```python
from build123d import *

# Parameters (mm, degrees)
SKETCH1_W           = 178
SKETCH1_H           = 104
SKETCH1_W_2         = 72
SKETCH1_H_2         = 68
BOSS_EXTRUDE1_DEPTH = 1.2
BOSS_EXTRUDE2_DEPTH = 5
SKETCH3_W           = 112
SKETCH3_H           = 10
BOSS_EXTRUDE3_DEPTH = 0.8
SKETCH4_W           = 10
SKETCH4_H           = 10
BOSS_EXTRUDE4_DEPTH = 2.8
SKETCH5_W           = 6
SKETCH5_H           = 2
CUT_EXTRUDE1_DEPTH  = 10
SKETCH6_W           = 10
SKETCH6_H           = 7.8
BOSS_EXTRUDE5_DEPTH = 6
FILLET1_R           = 10
FILLET2_R           = 6
SKETCH7_R           = 1.5
CUT_EXTRUDE2_DEPTH  = 4
FILLET3_R           = 3
SKETCH8_W           = 3
SKETCH8_H           = 10
BOSS_EXTRUDE6_DEPTH = 2.8
FILLET4_R           = 3
SKETCH9_W           = 10
SKETCH9_H           = 78
BOSS_EXTRUDE7_DEPTH = 2
BOSS_EXTRUDE8_DEPTH = 1.2


with BuildPart() as part:
    # Sketch1 → Boss-Extrude1 (new body)
    with BuildSketch(Plane(origin=(0, 0, 0), x_dir=(1, 0, 0), z_dir=(0, 1, 0))):
        with Locations((89, 52)):
            Rectangle(SKETCH1_W, SKETCH1_H)
        with Locations((126, 54)):
            Rectangle(SKETCH1_W_2, SKETCH1_H_2, mode=Mode.SUBTRACT)
        with Locations((44, 54)):
            Rectangle(SKETCH1_W_2, SKETCH1_H_2, mode=Mode.SUBTRACT)
    extrude(amount=BOSS_EXTRUDE1_DEPTH)

    # Sketch2 → Boss-Extrude2 (add)
    with BuildSketch(Plane(origin=(0, 0, -104), x_dir=(-1, 0, 0), z_dir=(0, 0, -1))):
        Polygon((-151, 0), (-148, 0), (-148, -2), (-144, -2), (-144, 0), (-141, 0), (-141, -4), (-144, -4), (-148, -4), (-151, -4), align=None)
    boss_extrude2 = extrude(amount=-BOSS_EXTRUDE2_DEPTH)

    # Mirror1: Boss-Extrude2 across plane
    add(boss_extrude2.mirror(Plane.ZY.offset(-78.75)))

    # Sketch3 → Boss-Extrude3 (add)
    with BuildSketch(Plane.XZ):
        with Locations((66, -10.2)):
            Rectangle(SKETCH3_W, SKETCH3_H)
    extrude(amount=BOSS_EXTRUDE3_DEPTH)

    # Sketch4 → Boss-Extrude4 (add)
    with BuildSketch(Plane.XZ):
        with Locations((5, -10.2)):
            Rectangle(SKETCH4_W, SKETCH4_H)
    extrude(amount=BOSS_EXTRUDE4_DEPTH)

    # Sketch5 → Cut-Extrude1 (cut)
    with BuildSketch(Plane.ZY):
        with Locations((-10.2, -1)):
            Rectangle(SKETCH5_W, SKETCH5_H)
    extrude(amount=-CUT_EXTRUDE1_DEPTH, mode=Mode.SUBTRACT)

    # Sketch6 → Boss-Extrude5 (add)
    with BuildSketch(Plane(origin=(0, 0, -104), x_dir=(-1, 0, 0), z_dir=(0, 0, -1))):
        with Locations((-89.25, -3.9)):
            Rectangle(SKETCH6_W, SKETCH6_H)
    extrude(amount=-BOSS_EXTRUDE5_DEPTH)

    # Fillet1
    # the kernel refuses this fillet: 10 mm, written as the material it adds along each edge
    with BuildSketch(Plane(origin=(94.25, 0, -104), x_dir=(1, 0, 0), z_dir=(0, 0, 1))) as fillet1_piece_1:
        with BuildLine():
            CenterArc((9.754998719, -10), FILLET1_R, 90, 77.290967006)
            Line((0, -7.8), (0, 0))
            Line((0, 0), (9.754998719, 0))
        make_face()
    extrude(amount=6)
    with BuildSketch(Plane(origin=(84.25, 0, -104), x_dir=(-1, 0, 0), z_dir=(0, 0, 1))) as fillet1_piece_2:
        with BuildLine():
            CenterArc((9.754998719, 10), FILLET1_R, 192.709032994, 77.290967006)
            Line((0, 7.8), (0, 0))
            Line((0, 0), (9.754998719, 0))
        make_face()
    extrude(amount=6)

    # Fillet2
    fillet2_edges = [part.edges().sort_by_distance(p)[0] for p in [
        (94.25, -7.8, -101),
        (84.25, -7.8, -101),
    ]]
    fillet(fillet2_edges, radius=FILLET2_R)

    # Sketch7 → Cut-Extrude2 (cut)
    with BuildSketch(Plane(origin=(0, 0, -104), x_dir=(-1, 0, 0), z_dir=(0, 0, -1))):
        with Locations((-89.25, -3.3)):
            Circle(SKETCH7_R)
    extrude(amount=-CUT_EXTRUDE2_DEPTH, mode=Mode.SUBTRACT)

    # Fillet3
    fillet3_edges = [part.edges().sort_by_distance(p)[0] for p in [
        (79.432105696, -1.303736435, -98),
        (99.067894304, -1.303736435, -98),
        (89.25, -7.8, -98),
        (85.271734229, -7.017758139, -98),
        (93.228265771, -7.017758139, -98),
    ]]
    fillet(fillet3_edges, radius=FILLET3_R)

    # Sketch8 → Boss-Extrude6 (add)
    with BuildSketch(Plane.XZ):
        with Locations((123.5, -10.2)):
            Rectangle(SKETCH8_W, SKETCH8_H)
    extrude(amount=BOSS_EXTRUDE6_DEPTH)

    # Fillet4
    # the kernel refuses this fillet: 3 mm, written as the material it adds along each edge
    with BuildSketch(Plane(origin=(125, 0, -5.2), x_dir=(1, 0, 0), z_dir=(0, 0, -1))) as fillet4_piece_1:
        with BuildLine():
            CenterArc((2.993325909, 3), FILLET4_R, 183.822553729, 86.177446271)
            Line((0, 2.8), (-0.059866518, 2.796))
            ThreePointArc((-0.059866518, 2.796), (-0.06, 1.4), (-0.06, 0))
            Line((-0.06, 0), (0, -0.06))
            Line((0, -0.06), (2.993325909, -0.06))
            Line((2.993325909, -0.06), (2.993325909, 0))
        make_face()
    extrude(amount=10)

    # Sketch9 → Boss-Extrude7 (add)
    with BuildSketch(Plane.XZ):
        with Locations((169, -39)):
            Rectangle(SKETCH9_W, SKETCH9_H)
    extrude(amount=BOSS_EXTRUDE7_DEPTH)

    # Sketch10 → Boss-Extrude8 (add)
    with BuildSketch(Plane(origin=(0, 1.2, 0), x_dir=(1, 0, 0), z_dir=(0, 1, 0))):
        with BuildLine():
            Line((15.496875383, 82.817231781), (37.139871313, 62.410978476))
            ThreePointArc((37.139871313, 62.410978476), (44, 59.686872538), (50.860128687, 62.410978476))
            Line((50.860128687, 62.410978476), (72.503124617, 82.817231781))
            ThreePointArc((72.503124617, 82.817231781), (73.233302704, 86.107180054), (70.445086011, 88))
            Line((70.445086011, 88), (53.755491102, 88))
            Line((53.755491102, 88), (53.755491102, 92.773114393))
            Line((53.755491102, 92.773114393), (83.607486332, 92.773114393))
            Line((83.607486332, 92.773114393), (83.607486332, 57.500394296))
            Line((83.607486332, 57.500394296), (80, 57.500394296))
            Line((80, 57.500394296), (80, 79.048223953))
            ThreePointArc((80, 79.048223953), (78.188672407, 81.802685408), (74.941961394, 81.230992171))
            Line((74.941961394, 81.230992171), (53.777463399, 61.275894062))
            ThreePointArc((53.777463399, 61.275894062), (50.637592086, 54), (53.777463399, 46.724105938))
            Line((53.777463399, 46.724105938), (74.941961394, 26.769007829))
            ThreePointArc((74.941961394, 26.769007829), (78.188672407, 26.197314592), (80, 28.951776047))
            Line((80, 28.951776047), (80, 51.757328614))
            Line((80, 51.757328614), (83.607486332, 51.757328614))
            Line((83.607486332, 51.757328614), (83.607486332, 17.03280878))
            Line((83.607486332, 17.03280878), (48.474442735, 17.03280878))
            Line((48.474442735, 17.03280878), (48.474442735, 20))
            Line((48.474442735, 20), (70.445086011, 20))
            ThreePointArc((70.445086011, 20), (73.233302704, 21.892819946), (72.503124617, 25.182768219))
            Line((72.503124617, 25.182768219), (50.860128687, 45.589021524))
            ThreePointArc((50.860128687, 45.589021524), (44, 48.313127462), (37.139871313, 45.589021524))
            Line((37.139871313, 45.589021524), (15.496875383, 25.182768219))
            ThreePointArc((15.496875383, 25.182768219), (14.766697296, 21.892819946), (17.554913989, 20))
            Line((17.554913989, 20), (45.016619204, 20))
            Line((45.016619204, 20), (45.016619204, 17.03280878))
            Line((45.016619204, 17.03280878), (3.455124081, 17.03280878))
            Line((3.455124081, 17.03280878), (3.455124081, 51.757328614))
            Line((3.455124081, 51.757328614), (8, 51.757328614))
            Line((8, 51.757328614), (8, 28.951776047))
            ThreePointArc((8, 28.951776047), (9.811327593, 26.197314592), (13.058038606, 26.769007829))
            Line((13.058038606, 26.769007829), (34.222536601, 46.724105938))
            ThreePointArc((34.222536601, 46.724105938), (37.362407914, 54), (34.222536601, 61.275894062))
            Line((34.222536601, 61.275894062), (13.058038606, 81.230992171))
            ThreePointArc((13.058038606, 81.230992171), (9.811327593, 81.802685408), (8, 79.048223953))
            Line((8, 79.048223953), (8, 56.332794756))
            Line((8, 56.332794756), (3.455124081, 56.332794756))
            Line((3.455124081, 56.332794756), (3.455124081, 92.773114393))
            Line((3.455124081, 92.773114393), (41.529538769, 92.773114393))
            Line((41.529538769, 92.773114393), (41.529538769, 88))
            Line((41.529538769, 88), (17.554913989, 88))
            ThreePointArc((17.554913989, 88), (14.766697296, 86.107180054), (15.496875383, 82.817231781))
        make_face()
    boss_extrude8 = extrude(amount=-BOSS_EXTRUDE8_DEPTH)

    # Mirror2: Boss-Extrude8 across plane
    add(boss_extrude8.mirror(Plane(origin=(85, 0, 0), x_dir=(0, 0, 1), z_dir=(1, 0, 0))))


solid = part.part
```
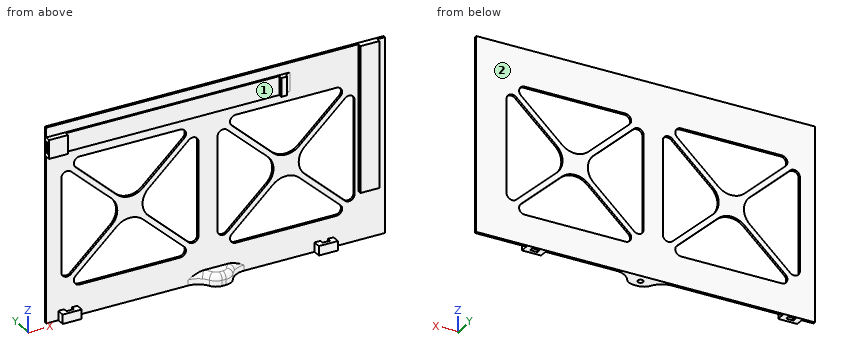
Model file for the job. Use its own axes, mm. Face numbers are marked on the shaded views. Coordinates: 2 decimals unless noted, no trailing zeros. Loops run counter-clockwise (first coordinate to the right, second up) from the corner with the lowest first, then second, coordinate; pieces in that order, holes last. Notation, with made-up numbers: (29.25, 31.5) - (82.25, 31.5) arc R34 cw to (82.25, 64.5) - close; hole circle Ø7 at (-21.75, 29.25). An arc over 180 degrees is marked (long way). Write item = value, one per line. Start each with the question number.
Item 1: Saw through at A-A, the plane x = 66. List the corners of the cut face in (y, z), then the cut area to 3 significant figures.
Item 2: Wall check: probe 1 along Y at (x, z) = (89, -102); probe 2 along Z at (x, y) = (24, -0.25); probe 3 along Z at (x, y) = (145, -3.75). Give the ranges that are in metal, low to high. Write a range as [from, to].
Item 3: Drop flat-ended pins along their axis: pin 1 Ø2 at (y, z) = (-1.5, -102.5) entering from -X; pin 2 Ø1.6 at (x, y) = (6, -1) entering from +Z; pin 3 Ø0.6 at (y, z) = (-1, -46) entering from +X; pin 4 Ø1.5 at (x, y) = (34.5, -2) entering from +Z. Give the stop position or say it passes through.
Item 4: Pull direction X, two halves, no side cores. Call the marked faces 1 and 2: +X half, -X half, draft (parallel to the pull), parting line (faces both ways), or undercut.
Answers:
q1.outline = (-0.8, -15.2) - (0, -15.2) - (0, -20) - (1.2, -20) - (1.2, 0) - (0, 0) - (0, -5.2) - (-0.8, -5.2) - close; (0, -104) - (1.2, -104) - (1.2, -88) - (0, -88) - close; (0, -76.69) - (1.2, -76.69) - (1.2, -72.8) - (0, -72.8) - close; (0, -35.2) - (1.2, -35.2) - (1.2, -31.31) - (0, -31.31) - close
q1.area = 60.5 mm2
q2.probe_1 = [-7.8, -4.78], [-1.82, 1.2]
q2.probe_2 = [-15.2, -5.2]
q2.probe_3 = [-104, -99]
q3.pin_1 = 6.5
q3.pin_2 = -5.2
q3.pin_3 = 174
q3.pin_4 = through
q4.face_1 = undercut
q4.face_2 = draft
